Design review of the part built by this model. Coordinates are the model's own, in mm. Face numbers are marked on the shaded views. Coordinates: 2 decimals unless noted, no trailing zeros. Loops run counter-clockwise (first coordinate to the right, second up) from the corner with the lowest first, then second, coordinate; pieces in that order, holes last. Notation, with made-up numbers: (1, -5.5) - (11, -5.5) arc R19 ccw to (11, 4.5) - close; hole circle Ø11 at (5.25, 39.5). An arc over 180 degrees is marked (long way). Answer in a Markdown table with one row per item. Add a question column.
(1) We need section D-D, the plane z = 4. Write out the cut boundary in (x, y), plus the area to 3 significant figures.
(2) We need section A-A, the plane x = 0. Write out the cut boundary in (y, z), plus the area to 3 significant figures.
(3) We need section B-B, the plane z = -3. Write out the cut boundary in (x, y).
(4) Clearance check with flat-ended pins moving along their axes: pin 1 (3 mm diameter, centred on y = -6, z = 4, fed in from -X); pin 2 (1.6 mm diameter, centred on y = 6, z = 4, fed in from -X); pin 3 (8.5 mm diameter, centred on x = 0, y = 0, fed in from +Z); pin 4 (0.9 mm diameter, centred on y = 6, z = 4, fed in from +X). State where each tip first meets the part, or that it passes through.
(5) To check wall thickness, follow L1, parallel to Z at x = -5, y = 6; L2, parallel to X at y = -7.6, z = 1.5; L3, parallel to X at y = 1.25, z = 8. State the ranges of each line that lie inside material, in increasing order. Write a range as [from, to].
(6) The part is to be moulded in two halves that separate along X. For the marked faces 1, 2, 3 and 4, say which applies: released by +X, released by -X, zero draft, split by the parting line, or undercut.
(7) We need section C-C, the plane y = 0. Write out the cut boundary in (x, z).
from build123d import *

# Parameters (mm, degrees)
SKETCH_1_W          = 16.3
SKETCH_1_H          = 20
SKETCH_1_R          = 5.25
EXTRUDE_1_DEPTH     = 10
SKETCH_1_6_W        = 16.3
SKETCH_1_6_H        = 20
EXTRUDE_2_DEPTH     = 2
SKETCH_2_R          = 0.9
CUT_EXTRUDE_1_DEPTH = 4
CUT_EXTRUDE_START   = -12.3
SKETCH_2_2_R        = 0.9
CUT_EXTRUDE_2_DEPTH = 4
SKETCH_3_W          = 5
SKETCH_3_H          = 20
EXTRUDE_3_DEPTH     = 16.3
SKETCH_5_R          = 0.9
CUT_EXTRUDE_3_DEPTH = 22.579851714
SKETCH_6_R          = 0.9
CUT_EXTRUDE_4_DEPTH = 4
CUT_EXTRUDE_START_2 = -16
SKETCH_6_3_R        = 0.9
CUT_EXTRUDE_5_DEPTH = 4


with BuildPart() as part:
    # 草图1 → 凸台-拉伸1 (new body)
    with BuildSketch(Plane.XY):
        Rectangle(SKETCH_1_W, SKETCH_1_H)
        Circle(SKETCH_1_R, mode=Mode.SUBTRACT)
    extrude(amount=EXTRUDE_1_DEPTH)

    # 草图1<6> → 凸台-拉伸2 (add)
    with BuildSketch(Plane.XY):
        Rectangle(SKETCH_1_6_W, SKETCH_1_6_H)
    extrude(amount=-EXTRUDE_2_DEPTH)

    # 草图2 → 切除-拉伸1 (cut)
    with BuildSketch(Plane.ZY.offset(8.15)):
        with Locations(Location((4, 6, 0), (0, 0, 270))):
            Circle(SKETCH_2_R)
        with Locations(Location((4, -6, 0), (0, 0, 270))):
            Circle(SKETCH_2_R)
    extrude(amount=-CUT_EXTRUDE_1_DEPTH, mode=Mode.SUBTRACT)

    # 草图2<2> → 切除-拉伸2 (cut)
    with BuildSketch(Plane.ZY.offset(8.15).offset(CUT_EXTRUDE_START)):
        with Locations(Location((4, 6, 0), (0, 0, 270))):
            Circle(SKETCH_2_2_R)
        with Locations(Location((4, -6, 0), (0, 0, 270))):
            Circle(SKETCH_2_2_R)
    extrude(amount=-CUT_EXTRUDE_2_DEPTH, mode=Mode.SUBTRACT)

    # 草图3 → 凸台-拉伸3 (add)
    with BuildSketch(Plane(origin=(8.15, 0, 0), x_dir=(0, 0, -1), z_dir=(1, 0, 0))):
        with Locations((4.5, 0)):
            Rectangle(SKETCH_3_W, SKETCH_3_H)
    extrude(amount=-EXTRUDE_3_DEPTH)

    # 草图5 → 切除-拉伸3 (cut, through all)
    with BuildSketch(Plane.ZY.offset(8.15)):
        with Locations(Location((-3, 0, 0), (0, 0, 270))):
            Circle(SKETCH_5_R)
    extrude(amount=-CUT_EXTRUDE_3_DEPTH, mode=Mode.SUBTRACT)

    # 草图6 → 切除-拉伸4 (cut)
    with BuildSketch(Plane.XZ.offset(10)):
        with Locations(Location((0, 1.5, 0), (0, 0, 270))):
            Circle(SKETCH_6_R)
    extrude(amount=-CUT_EXTRUDE_4_DEPTH, mode=Mode.SUBTRACT)

    # 草图6<3> → 切除-拉伸5 (cut)
    with BuildSketch(Plane.XZ.offset(10).offset(CUT_EXTRUDE_START_2)):
        with Locations(Location((0, 1.5, 0), (0, 0, 270))):
            Circle(SKETCH_6_3_R)
    extrude(amount=-CUT_EXTRUDE_5_DEPTH, mode=Mode.SUBTRACT)


solid = part.part
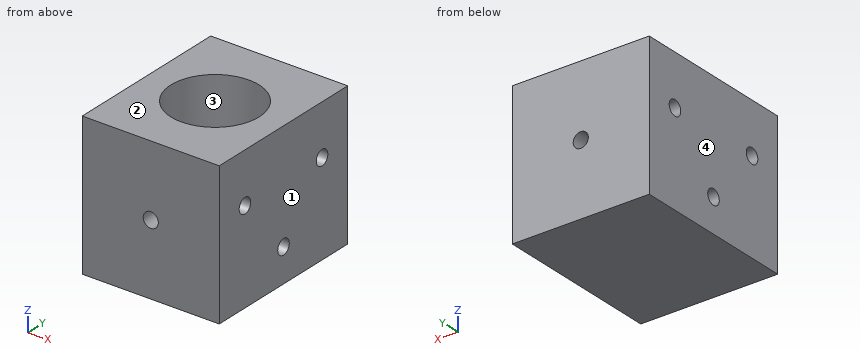
Responses:
| question | item | result |
|---|---|---|
| 1 | outline | (-8.15, -10) - (8.15, -10) - (8.15, -6.9) - (4.15, -6.9) - (4.15, -5.1) - (8.15, -5.1) - (8.15, 5.1) - (4.15, 5.1) - (4.15, 6.9) - (8.15, 6.9) - (8.15, 10) - (-8.15, 10) - (-8.15, 6.9) - (-4.15, 6.9) - (-4.15, 5.1) - (-8.15, 5.1) - (-8.15, -5.1) - (-4.15, -5.1) - (-4.15, -6.9) - (-8.15, -6.9) - close; hole circle Ø10.5 at (0, 0) |
| 1 | area | 211 mm2 |
| 2 | outline | (-10, -7) - (10, -7) - (10, 0.6) - (6, 0.6) - (6, 2.4) - (10, 2.4) - (10, 10) - (5.25, 10) - (5.25, 0) - (-5.25, 0) - (-5.25, 10) - (-10, 10) - (-10, 2.4) - (-6, 2.4) - (-6, 0.6) - (-10, 0.6) - close; hole circle Ø1.8 at (0, -3) |
| 2 | area | 218 mm2 |
| 3 | outline | (-8.15, -10) - (8.15, -10) - (8.15, -0.9) - (-8.15, -0.9) - close; (-8.15, 0.9) - (8.15, 0.9) - (8.15, 10) - (-8.15, 10) - close |
| 4 | pin 1 | stops at x = -8.15 |
| 4 | pin 2 | stops at x = -4.15 |
| 4 | pin 3 | stops at z = 0 |
| 4 | pin 4 | stops at x = 4.15 |
| 5 | L1 | z = [-7, 3.1], [4.9, 10] |
| 5 | L2 | x = [-8.15, -0.9], [0.9, 8.15] |
| 5 | L3 | x = [-8.15, -5.1], [5.1, 8.15] |
| 6 | face 1 | released by +X |
| 6 | face 2 | zero draft |
| 6 | face 3 | undercut |
| 6 | face 4 | released by -X |
| 7 | outline | (-8.15, -7) - (8.15, -7) - (8.15, -3.9) - (-8.15, -3.9) - close; (-8.15, -2.1) - (8.15, -2.1) - (8.15, 10) - (5.25, 10) - (5.25, 0) - (-5.25, 0) - (-5.25, 10) - (-8.15, 10) - close |
